```python
from build123d import *

# Parameters (mm, degrees)
SKETCH1_R           = 3.81
SKETCH1_R_2         = 3.429
BOSS_EXTRUDE1_DEPTH = 10.16
SKETCH2_W           = 88.9
SKETCH2_H           = 65.208376681
BOSS_EXTRUDE2_DEPTH = 12.7
CUT_EXTRUDE1_START  = -12.7
SKETCH1_3_R         = 3.429
CUT_EXTRUDE1_DEPTH  = 12.7


with BuildPart() as part:
    # Sketch1 → Boss-Extrude1 (new body)
    with BuildSketch(Plane.XY):
        Polygon((0, 0), (38.1, 0), (63.5, 127), (63.5, 190.5), (-25.4, 190.5), (-25.4, 125.291623319), align=None)
        with Locations((19.05, 12.7)):
            Circle(SKETCH1_R, mode=Mode.SUBTRACT)
        with Locations((19.05, 50.8)):
            Circle(SKETCH1_R, mode=Mode.SUBTRACT)
        with Locations((-6.35, 174.687730396)):
            Circle(SKETCH1_R_2, mode=Mode.SUBTRACT)
        with Locations((-6.35, 149.287730396)):
            Circle(SKETCH1_R_2, mode=Mode.SUBTRACT)
        with Locations(Location((44.45, 149.287730396, 0), (0, 0, 180))):
            Circle(SKETCH1_R_2, mode=Mode.SUBTRACT)
        with Locations(Location((44.45, 174.687730396, 0), (0, 0, 180))):
            Circle(SKETCH1_R_2, mode=Mode.SUBTRACT)
    extrude(amount=BOSS_EXTRUDE1_DEPTH)

    # Sketch2 → Boss-Extrude2 (add)
    with BuildSketch(Plane(origin=(0, 0, 0), x_dir=(-1, 0, 0), z_dir=(0, 0, -1))):
        with Locations((-19.05, 157.895811659)):
            Rectangle(SKETCH2_W, SKETCH2_H)
    extrude(amount=BOSS_EXTRUDE2_DEPTH)

    # Sketch1<3> → Cut-Extrude1 (cut)
    with BuildSketch(Plane.XY.offset(CUT_EXTRUDE1_START)):
        with Locations(Location((-6.35, 174.687730396, 0), (0, 0, 180))):
            Circle(SKETCH1_3_R)
        with Locations(Location((-6.35, 149.287730396, 0), (0, 0, 180))):
            Circle(SKETCH1_3_R)
        with Locations(Location((44.45, 149.287730396, 0), (0, 0, 180))):
            Circle(SKETCH1_3_R)
        with Locations(Location((44.45, 174.687730396, 0), (0, 0, 180))):
            Circle(SKETCH1_3_R)
    extrude(amount=CUT_EXTRUDE1_DEPTH, mode=Mode.SUBTRACT)


solid = part.part
```
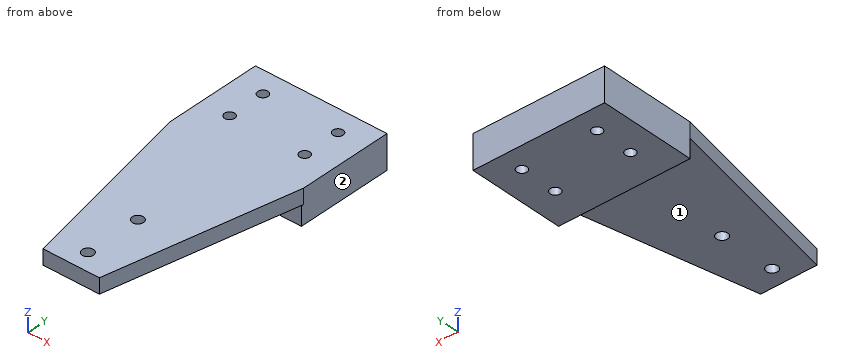
Model file for the job. Use its own axes, mm. Face numbers are marked on the shaded views. A direction names the side the tool comes from. Round coordinates to 2 decimals unless told otherwise and drop trailing zeros. Write each loop counter-clockwise with the first axis right and the second up, starting at its lowest first coordinate (ties: lowest second). Pieces come first, ordered by that corner, then holes. Notation, with made-up numbers: M 4.5,89.5 L 47.5,89.5 A29 cw 47.5,115.5 Z; hole C -12,77.25 d2. An arc over 180 degrees is marked long. Put each result on its own line as item: value.
Item 1: Probe L1, parallel to Y at x = 19.05, z = 5; L2, parallel to X at y = 173.5, z = 1.5; L3, parallel to Y at x = 42.5, z = -2.75. List the from-to ranges inside material, lowest first. Write a range as from..to.
Responses:
L1: 0..8.89, 16.51..46.99, 54.61..190.5
L2: -25.4..-9.57, -3.13..41.23, 47.67..63.5
L3: 125.29..146.47, 152.11..171.87, 177.51..190.5
Item 2: Tool access for the marked faces 1 and 2: list every direction of +Z, -Z, +X, -X, +Y, -Y with a clear straight run to the whole face (end or side of a thin tool).
Responses:
face 1: -Z, +X, -X, -Y
face 2: +Z, -Z, +X, +Y, -Y
Item 3: Cut at B-B (z = -9.5). List the corners of the cut face in (x, y).
Responses:
outline: M -25.4,125.29 L 63.5,125.29 L 63.5,190.5 L -25.4,190.5 Z; hole C -6.35,149.29 d6.86; hole C -6.35,174.69 d6.86; hole C 44.45,149.29 d6.86; hole C 44.45,174.69 d6.86
Item 4: Cut at A-A (x = 44.45). List the corners of the cut face in (y, z), and give its area (3 significant figures).
Responses:
outline: M 31.75,0 L 125.29,0 L 125.29,-12.7 L 145.86,-12.7 L 145.86,10.16 L 31.75,10.16 Z; M 152.72,-12.7 L 171.26,-12.7 L 171.26,10.16 L 152.72,10.16 Z; M 178.12,-12.7 L 190.5,-12.7 L 190.5,10.16 L 178.12,10.16 Z
area: 2,130 mm²
Item 5: Cut at D-D (x = 13). List the corners of the cut face in (y, z), and give its area (3 significant figures).
Responses:
outline: M 0,0 L 125.29,0 L 125.29,-12.7 L 190.5,-12.7 L 190.5,10.16 L 0,10.16 Z
area: 2,760 mm²
Item 6: Cut at C-C (y = 12.7). List the corners of the cut face in (x, z), and give its area (3 significant figures).
Responses:
outline: M -2.57,0 L 15.24,0 L 15.24,10.16 L -2.57,10.16 Z; M 22.86,0 L 40.64,0 L 40.64,10.16 L 22.86,10.16 Z
area: 362 mm²
Item 7: Flat gauge pins, fed straight in: P1, Ø9, axis at x = -6.35, y = 149.29, coming from the -Z side; P2, Ø4, axis at x = 44.45, y = 174.69, coming from the +Z side; P3, Ø2, axis at x = 31.5, z = -2, coming from the -Y side; P4, Ø8, axis at y = 91, z = -0.5, coming from the +X side. Where does each tip first touch, or does it go through?
Responses:
P1: z = -12.7
P2: through
P3: y = 125.29
P4: x = 57.09
